Autodesk Inventor part; units mm, degrees
ref_plane "to_collar_XY" through (449, 0, 0) normal (1, 0, 0) x (0, 0, -1)
ref_plane "to_collar_YZ" through (449, 0, 0) normal (0, 0, -1) x (0, 1, 0)
ref_plane "to_collar_ZX" through (449, 0, 0) normal (0, 1, 0) x (1, 0, 0)
sketch "Sketch_1" plane through (0, 0, 0) normal (0, 0, 1) x (1, 0, 0)
  line L0 (449.5, 0) -> (0, 0)
  line L1 (0, 0) -> (0, 3.5)
  line L2 (0, 3.5) -> (0.5, 4)
  line L3 (0.5, 4) -> (2.1, 4)
  line L4 (2.1, 4) -> (2.1, 3.8)
  line L5 (2.1, 3.8) -> (3, 3.8)
  line L6 (3, 3.8) -> (3, 4)
  line L7 (3, 4) -> (9.5, 4)
  arc A0 (9.5, 4) -> (10, 4.5) centre (9.5, 4.5) ccw
  line L8 (10, 4.5) -> (10, 5.5)
  line L9 (10, 5.5) -> (10.5, 6)
  line L10 (10.5, 6) -> (448.5, 6)
  line L11 (448.5, 6) -> (449, 5.5)
  arc A1 (449, 5.5) -> (449.5, 5) centre (449.5, 5.5) ccw
  line L12 (449.5, 5) -> (449.5, 0)
  line L13 (449.5, 0) -> (0, 0)
revolve "Revolution1" add sketch "Sketch_1" angle 360 about axis through (449.5, 0, 0) along (1, 0, 0)
thread "Thread1"
sketch "_____2" plane through (0, 0, 0) normal (0, 0, 1) x (1, 0, 0)
  line L0 (500, 0) -> (449.5, 0)
  line L1 (449.5, 0) -> (449.5, 5)
  line L2 (449.5, 5) -> (484.5, 5)
  line L3 (484.5, 5) -> (485, 4.5)
  line L4 (485, 4.5) -> (485, 4.3)
  arc A0 (485, 4.3) -> (485.3, 4) centre (485.3, 4.3) ccw
  line L5 (485.3, 4) -> (499.5, 4)
  line L6 (499.5, 4) -> (500, 3.5)
  line L7 (500, 3.5) -> (500, 0)
  line L8 (500, 0) -> (449.5, 0)
revolve "Revolution2" add sketch "_____2" angle 360 about axis through (500, 0, 0) along (1, 0, 0)
thread "Thread2"
ref_plane "to_collar_XY" through (449, 0, 0) normal (1, 0, 0) x (0, 0, -1)
ref_plane "to_collar_YZ" through (449, 0, 0) normal (0, 0, -1) x (0, 1, 0)
ref_plane "to_collar_ZX" through (449, 0, 0) normal (0, 1, 0) x (1, 0, 0)
ref_plane "to_dummy_XY" through (10, 0, 0) normal (1, 0, 0) x (0, 0, -1)
ref_plane "to_dummy_YZ" through (10, 0, 0) normal (0, 0, -1) x (0, 1, 0)
ref_plane "to_dummy_ZX" through (10, 0, 0) normal (0, 1, 0) x (1, 0, 0)
ref_plane "to_nut_XY" through (229.5, 0, 0) normal (1, 0, 0) x (0, 0, -1)
ref_plane "to_nut_YZ" through (229.5, 0, 0) normal (0, 0, -1) x (0, 1, 0)
ref_plane "to_nut_ZX" through (229.5, 0, 0) normal (0, 1, 0) x (1, 0, 0)
properties part number "C-TBSE1204-500_t"
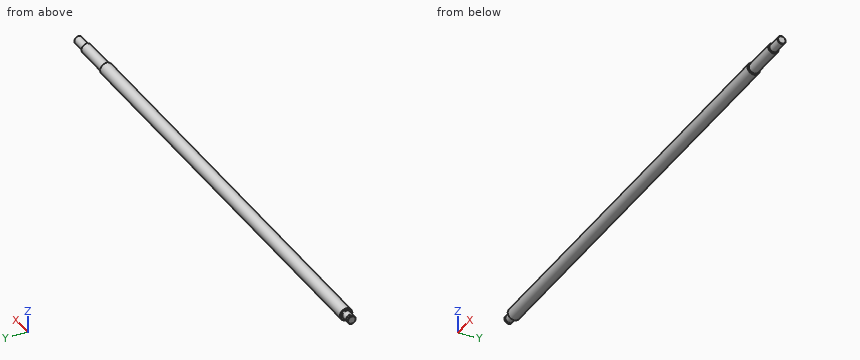
Could you check a few things on this model? Use its own coordinates, in mm. Give positions to 0.01 mm unless a question says otherwise; leave off trailing zeros. Write each loop counter-clockwise with the first axis right and the second up, starting at its lowest first coordinate (ties: lowest second). Pieces come first, ordered by that corner, then holes. Notation, with made-up numbers: (52, 1) - (82, 1) arc R22 ccw to (82, 31) - close; hole circle Ø7 at (9.25, 26). An arc over 180 degrees is marked (long way). One line per item, written item: value. Start each with the question number.
Item 1: I'm going to push flat-ended pins straight in: pin 1 (1 mm diameter, centred on x = 388, y = 4.5, fed in from +Z); pin 2 (1 mm diameter, centred on x = 339, y = 1.5, fed in from -Z). Where does each tip first touch, or does it pass through?
Item 2: Please list where these lines run through material, in increasing order: line 1 (Z direction, x = 384.5, y = -4); line 2 (Z direction, x = 233.5, y = 1); line 3 (X direction, y = 3.25, z = 1.5). Write a range as from..to.
Item 3: Imagine slicing it at A-A, the plane x = 191.5. List the corners of the cut face in (y, z) for me.
Geometry says:
1. pin 1: z = 4.47
1. pin 2: z = -5.92
2. line 1: -4.47..4.47
2. line 2: -5.92..5.92
2. line 3: 0.08..499.92
3. outline: circle Ø12 at (0, 0)
